from build123d import *

# Parameters (mm, degrees)
F0_R     = 69.2237369755
F1_DEPTH = 50.8
F2_SIZE  = 5.08
F3_DEPTH = 25.4
F4_SIZE  = 5.08
F5_DEPTH = 25.4
F6_SIZE  = 5.08
F7_DEPTH = 50.8


with BuildPart() as f1:
    # F0 (on Front) → F1 (new body)
    with BuildSketch(Plane.XZ):
        with Locations((-16.0285290331, 36.5865901113)):
            Circle(F0_R)
    extrude(amount=F1_DEPTH)

    # F2
    f2_edges = [f1.edges().sort_by_distance(p)[0] for p in [
        (53.195208, -25.4, 36.58659),
        (-85.252266, 0, 36.58659),
        (-85.252266, -50.8, 36.58659),
    ]]
    chamfer(f2_edges, length=F2_SIZE)

    # F3 (add): a face of the model
    f3_faces = [f1.faces().sort_by_distance(p)[0] for p in [
        (-16.0285290331, -50.8, 36.5865901113),
    ]]
    extrude(f3_faces, amount=F3_DEPTH)

    # F4
    f4_edges = [f1.edges().sort_by_distance(p)[0] for p in [
        (-80.172266, -76.2, 36.58659),
    ]]
    chamfer(f4_edges, length=F4_SIZE)

    # F5 (add): a face of the model
    f5_faces = [f1.faces().sort_by_distance(p)[0] for p in [
        (-16.0285290331, -76.2, 36.5865901113),
    ]]
    extrude(f5_faces, amount=F5_DEPTH)

    # F6
    f6_edges = [f1.edges().sort_by_distance(p)[0] for p in [
        (-75.092266, -101.6, 36.58659),
    ]]
    chamfer(f6_edges, length=F6_SIZE)

    # F7 (add): a face of the model
    f7_faces = [f1.faces().sort_by_distance(p)[0] for p in [
        (-16.0285290331, -101.6, 36.5865901113),
    ]]
    extrude(f7_faces, amount=F7_DEPTH)


solid = f1.part
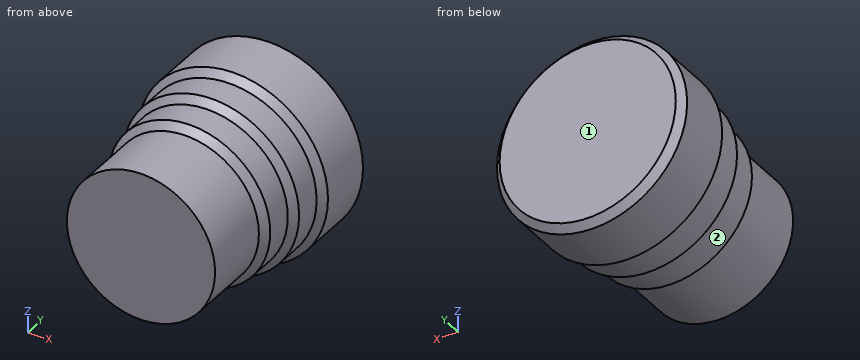
Geometry check sheet. Reference: the model listing, model coordinates, mm. Face numbers are marked on the shaded views. A direction names the side the tool comes from. Round coordinates to 2 decimals unless told otherwise and drop trailing zeros. Order: outer loops, then holes, each group sorted by start corner. A loop starts at its lowest first (then second) coordinate and runs counter-clockwise, first axis right, second up. Notation, with made-up numbers: (15.25, -12.75) - (28.25, -12.75) arc R27 ccw to (28.25, 19.25) - close; hole circle Ø5 at (71, -28). An arc over 180 degrees is marked (long way). One line per question, with ' | ' between items. Start each with the question number.
(1) Access from +Z, -Z, +X, -X, +Y, -Y to the whole of each face (thin tool, end or side, straight path). Record for the marked faces 1 and 2.
(2) Depth check by flat-ended pin: pin 1 Ø1.5 at (x, y) = (-32.5, -113) entering from +Z; pin 2 Ø10 at (y, z) = (-48.5, -7.5) entering from +X; pin 3 Ø6 at (x, y) = (-54, -60) entering from -Z. Enter the tip coordinate at first touch or a pass-through.
(3) Thickness scan on L1, parallel to Z at x = -17.5, y = -84; L2, parallel to X at y = -18.5, z = 39.5; L3, parallel to Z at x = -14, y = -17.5. Record the ranges inside material, lowest first. Write a range as [from, to].
(4) Sectioned sample at A-A on y = -99. Record the cut outline in (x, z).
(5) Sectioned sample at B-B on y = -135. Record the cut outline in (x, z), and give its area (3 significant figures).
Conclusion:
1) face 1: +Z, -Z, +X, -X, +Y | face 2: -Y
2) pin 1: stops at z = 88.23 | pin 2: stops at x = 40.52 | pin 3: stops at z = -17.19
3) L1: z = [-22.46, 95.63] | L2: x = [-85.19, 53.13] | L3: z = [-32.61, 105.78]
4) outline: circle Ø113.17 at (-16.03, 36.59)
5) outline: circle Ø107.97 at (-16.03, 36.59) | area: 9,160 mm2
